The model under review builds one solid part; all positions refer to its coordinate system, in mm. A direction names the side the tool comes from. Coordinates: 2 decimals unless noted, no trailing zeros. Loops run counter-clockwise (first coordinate to the right, second up) from the corner with the lowest first, then second, coordinate; pieces in that order, holes last. Notation, with made-up numbers: (45.25, 74) - (52.25, 74) arc R22 cw to (52.25, 93) - close; hole circle Ø8 at (16, 22). An arc over 180 degrees is marked (long way). Use a Markdown table: item, result. Add a question column.
1) Clearance check with flat-ended pins moving along their axes: pin 1 (6 mm diameter, centred on x = 146.5, z = -19, fed in from -Y); pin 2 (8 mm diameter, centred on y = 299.5, z = -6.5, fed in from -X); pin 3 (10 mm diameter, centred on x = 116.5, z = -10.5, fed in from +Y). State where each tip first meets the part, or that it passes through.
2) Add section B-B, the plane y = -77. Give the boundary of the cut face in (x, z), and give its area (3 significant figures).
3) Add section A-A, the plane x = -68. Give the boundary of the cut face in (y, z), and give its area (3 significant figures).
4) To check wall thickness, follow L1, parallel to Y at x = 30, z = -51.5; L2, parallel to Y at x = -62, z = -12.5; L3, parallel to X at y = 206.5, z = -13.5. State the ranges of each line that lie inside material, in increasing order. Write a range as [from, to].
5) The part is to be moulded in two halves that separate along Y. For faces 6 (the flat face through (2, -331, -25)), 7 (the flat face through (2, 325, -28)), 8 (the flat face through (156, -5, -25)), say which applies: pulls with the +Y half, pulls with the -Y half, needs draft (parallel to the pull), parting line crosses it, or undercut.
6) Add section C-C, the plane z = -8. Give the boundary of the cut face in (x, y), and give its area (3 significant figures).
7) For faces 1 (the flat face through (2, 331, -25)), 2 (the flat face through (2, -325, -28)), 3 (the flat face through (151, -2, 0)), 4 (the flat face through (-156, -5, -25)), 5 (the flat face through (180, -5, -56)), list the 3-axis set-ups (+Z, -Z, +X, -X, +Y, -Y) from which the entire face can be reached by the end or side of a thin tool; tool diameter is ignored.
```python
from build123d import *

# Parameters (mm, degrees)
SKETCH054_W            = 300
SKETCH054_H            = 60
PAD003_DEPTH           = 325
SKETCH004_W            = 312
SKETCH004_H            = 50
PAD004_DEPTH           = 331
SKETCH055_W            = 412
SKETCH055_H            = 762
PAD005_DEPTH           = 6
CUT001_PLACEMENT_ANGLE = 180


with BuildPart() as body002:
    # Sketch054 → Pad003 (new body, symmetric)
    with BuildSketch(Plane.XZ):
        with Locations((0, 30)):
            Rectangle(SKETCH054_W, SKETCH054_H)
    extrude(amount=PAD003_DEPTH, both=True)


with BuildPart() as cut001:
    # Sketch004 → Pad004 (new body, symmetric)
    with BuildSketch(Plane.XZ):
        with Locations((0, 25)):
            Rectangle(SKETCH004_W, SKETCH004_H)
    extrude(amount=PAD004_DEPTH, both=True)

    # Sketch055 (on Face3 of Pad004) → Pad005 (join)
    with BuildSketch(Plane(origin=(0, 0, 50), x_dir=(-1, 0, 0), z_dir=(0, 0, 1))):
        Rectangle(SKETCH055_W, SKETCH055_H)
    extrude(amount=PAD005_DEPTH)

    # Cut001: cut Body002
    add(body002.part, mode=Mode.SUBTRACT)


with BuildPart() as cut001_1:
    # Cut001 placement: moved
    add(cut001.part.rotate(Axis((0, 0, 0), (0, 1, 0)), CUT001_PLACEMENT_ANGLE))


solid = cut001_1.part
```
From the geometry:
| question | item | result |
|---|---|---|
| 1 | pin 1 | stops at y = -331 |
| 1 | pin 2 | stops at x = -156 |
| 1 | pin 3 | stops at y = 331 |
| 2 | outline | (-206, -56) - (-150, -56) - (-150, 0) - (-156, 0) - (-156, -50) - (-206, -50) - close; (150, -56) - (206, -56) - (206, -50) - (156, -50) - (156, 0) - (150, 0) - close |
| 2 | area | 1,270 mm^2 |
| 3 | outline | (-381, -56) - (-325, -56) - (-325, 0) - (-331, 0) - (-331, -50) - (-381, -50) - close; (325, -56) - (381, -56) - (381, -50) - (331, -50) - (331, 0) - (325, 0) - close |
| 3 | area | 1,270 mm^2 |
| 4 | L1 | y = [-381, -325], [325, 381] |
| 4 | L2 | y = [-331, -325], [325, 331] |
| 4 | L3 | x = [-156, -150], [150, 156] |
| 5 | face 6 | pulls with the -Y half |
| 5 | face 7 | undercut |
| 5 | face 8 | needs draft |
| 6 | outline | (-156, -331) - (156, -331) - (156, 331) - (-156, 331) - close; hole (-150, -325) - (150, -325) - (150, 325) - (-150, 325) - close |
| 6 | area | 11,500 mm^2 |
| 7 | face 1 | +Z, +X, -X, +Y |
| 7 | face 2 | +Z, -Z |
| 7 | face 3 | +Z, +X, -X, +Y, -Y |
| 7 | face 4 | +Z, -X, +Y, -Y |
| 7 | face 5 | -Z, +X, -X, +Y, -Y |
